from build123d import *

# Parameters (mm, degrees)
SKETCH1_W           = 55.5
SKETCH1_H           = 43.2
BASE_DEPTH          = 5
SKETCH2_W           = 55.5
SKETCH2_H           = 25.5
WALL_DEPTH          = 5
SKETCH3_W           = 7
SKETCH3_H           = 20.5
MOUNTINGTABS_DEPTH  = 5
LIPS_REACH          = 76.811
SKETCH5_R           = 1.75
MOUNTINGHOLES_DEPTH = 5
FILLETS_R           = 3.5
SKETCH6_R           = 1.75
THROUGHHOLE_DEPTH   = 5


with BuildPart() as part:
    # Sketch1 → base (new body)
    with BuildSketch(Plane(origin=(0, 0, 0), x_dir=(1, 0, 0), z_dir=(0, 1, 0))):
        with Locations((27.75, 21.6)):
            Rectangle(SKETCH1_W, SKETCH1_H)
    extrude(amount=BASE_DEPTH)

    # Sketch2 → wall (add)
    with BuildSketch(Plane(origin=(0, 0, -43.2), x_dir=(-1, 0, 0), z_dir=(0, 0, -1))):
        with Locations((-27.75, 12.75)):
            Rectangle(SKETCH2_W, SKETCH2_H)
    extrude(amount=-WALL_DEPTH)

    # Sketch3 → mountingTabs (add)
    with BuildSketch(Plane.XY.offset(-8.2)):
        with Locations((3.5, 15.25)):
            Rectangle(SKETCH3_W, SKETCH3_H)
        with Locations((52, 15.25)):
            Rectangle(SKETCH3_W, SKETCH3_H)
    extrude(amount=MOUNTINGTABS_DEPTH)

    # lips: up to this face of the body (flat: up to its plane)
    lips_end = Plane(part.part.faces().sort_by_distance((27.75, 12.75, -43.2))[0])
    # Sketch4 → lips (add, up to the picked face)
    with BuildSketch(Plane.XY, mode=Mode.PRIVATE) as lips_sk1:
        with BuildLine():
            Line((0, 0), (-10.208884478, 7.148337868))
            ThreePointArc((-10.208884478, 7.148337868), (-11.894564223, 9.792816133), (-11.218174515, 12.85505036))
            Line((-11.218174515, 12.85505036), (0, 5))
            Line((0, 5), (0, 0))
        make_face()
    lips_tool1 = split(extrude(lips_sk1.sketch, amount=-LIPS_REACH, mode=Mode.PRIVATE), bisect_by=lips_end, keep=Keep.BOTH, mode=Mode.PRIVATE)
    # Sketch4 → lips (add, up to the picked face)
    with BuildSketch(Plane.XY, mode=Mode.PRIVATE) as lips_sk2:
        with BuildLine():
            Line((55.5, 5), (66.718174515, 12.85505036))
            ThreePointArc((66.718174515, 12.85505036), (67.394564223, 9.792816133), (65.708884478, 7.148337868))
            Line((65.708884478, 7.148337868), (55.5, 0))
            Line((55.5, 0), (55.5, 5))
        make_face()
    lips_tool2 = split(extrude(lips_sk2.sketch, amount=-LIPS_REACH, mode=Mode.PRIVATE), bisect_by=lips_end, keep=Keep.BOTH, mode=Mode.PRIVATE)
    add(lips_tool1.solids().sort_by(Axis((-5.839287, 6.590277, 0), (0, 0, -1)))[0])
    add(lips_tool2.solids().sort_by(Axis((61.339287, 6.590277, 0), (0, 0, -1)))[0])

    # Sketch5 → mountingHoles (cut)
    with BuildSketch(Plane.XY.offset(-3.2)):
        with Locations((3.75, 20.25)):
            Circle(SKETCH5_R)
        with Locations(Location((3.75, 10.25, 0), (0, 0, 180))):
            Circle(SKETCH5_R)
        with Locations((51.75, 10.25)):
            Circle(SKETCH5_R)
        with Locations(Location((51.75, 20.25, 0), (0, 0, 180))):
            Circle(SKETCH5_R)
    extrude(amount=-MOUNTINGHOLES_DEPTH, mode=Mode.SUBTRACT)

    # fillets
    fillets_edges = [part.edges().sort_by_distance(p)[0] for p in [
        (0, 25.5, -40.7),
        (55.5, 25.5, -40.7),
        (0, 25.5, -5.7),
        (55.5, 25.5, -5.7),
    ]]
    fillet(fillets_edges, radius=FILLETS_R)

    # Sketch6 → throughHole (cut)
    with BuildSketch(Plane.XY.offset(-38.2)):
        with Locations((38.25, 15.25)):
            Circle(SKETCH6_R)
    extrude(amount=-THROUGHHOLE_DEPTH, mode=Mode.SUBTRACT)


solid = part.part
The listing builds one solid part. Answer for the finished solid, in the listing's coordinates (mm). A direction names the side the tool comes from. Round coordinates to 2 decimals unless told otherwise and drop trailing zeros. Loops run counter-clockwise (first coordinate to the right, second up) from the corner with the lowest first, then second, coordinate; pieces in that order, holes last. Notation, with made-up numbers: M -39.75,17 L -1.75,17 A26 cw -1.75,55 Z; hole C 4,-27.5 d7. An arc over 180 degrees is marked long. Write each question's results on one line, items separated by ' | '. Start each with the question number.
1) Which of the six approach directions +Z, -Z, +X, -X, +Y, -Y give full straight-line access (tool end or side, diameter ignored) to faces 1 (the flat face through (50, 25.5, -6)), 2 (the flat face through (-5.688, 8.983, -21.298)), 3 (the flat face through (48.5, 15, -6)), 4 (the cylindrical face through (50.081, 19.724, -5.665)), 5 (the flat face through (28, 15, -38.2))?
2) Each of these flat-tipped pins is pushed along its axis until it touches: pin 1 (5.5 mm diameter, centred on y = 19, z = -5.5, fed in from +X); pin 2 (5.5 mm diameter, centred on x = 50.5, y = 15, fed in from +Z); pin 3 (3 mm diameter, centred on y = 4.5, z = -14, fed in from -X). Where does it stop, or does it pass through?
3) Find section D-D on x = 47.5. Write down the section's boundary in (y, z).
4) Find section C-C on z = -14.5. Write down the section's boundary in (x, y).
5) Determine the mould class of faces 6 (the flat face through (0, 13, -41)), 7 (the cylindrical face through (1, 24.45, -5.66)), 8 (the flat face through (28, 25.5, -41)) for opening direction X: pulls with the +X half, pulls with the -X half, needs draft (parallel to the pull), parting line crosses it, or undercut.
6) Find section B-B on y = 15.25. Write down the section's boundary in (x, z).
7) Find section A-A on x = 38.25. Write down the section's boundary in (y, z), plus the area to 3 significant figures.
8) Straight lines are drawn through the part: probe 1 along Y at (x, z) = (3.75, -4.85); probe 2 along Z at (x, y) = (54.5, 15); probe 3 along X at (y, z) = (15, -39.5). For each, find the intervals that lie inside material, in ascending order.
Final values:
1) face 1: +Z, -Z, +X, -X, +Y | face 2: +Z, -Z, +Y | face 3: +Z, +Y | face 4: +Z | face 5: +Y
2) pin 1: x = 55.5 | pin 2: z = -3.2 | pin 3: x = -8.57
3) outline: M 0,-43.2 L 25.5,-43.2 L 25.5,-38.2 L 5,-38.2 L 5,0 L 0,0 Z
4) outline: M -11.22,12.86 A4.1 ccw -10.21,7.15 L 0,0 L 55.5,0 L 65.71,7.15 A4.1 ccw 66.72,12.86 L 55.5,5 L 0,5 Z
5) face 6: undercut | face 7: pulls with the -X half | face 8: needs draft
6) outline: M 0,-43.2 L 36.5,-43.2 L 36.5,-38.2 L 0,-38.2 Z; M 0,-8.2 L 7,-8.2 L 7,-3.2 L 0,-3.2 Z; M 40,-43.2 L 55.5,-43.2 L 55.5,-38.2 L 40,-38.2 Z; M 48.5,-8.2 L 55.5,-8.2 L 55.5,-3.2 L 48.5,-3.2 Z
7) outline: M 0,-43.2 L 13.5,-43.2 L 13.5,-38.2 L 5,-38.2 L 5,0 L 0,0 Z; M 17,-43.2 L 25.5,-43.2 L 25.5,-38.2 L 17,-38.2 Z | area: 301 mm²
8) probe 1: 0 to 8.5, 12 to 18.5, 22 to 25.5 | probe 2: -43.2 to -38.2, -8.2 to -3.2 | probe 3: 0 to 36.52, 39.98 to 55.5
